The model under review builds one solid part; all positions refer to its coordinate system, in mm. Round coordinates to 2 decimals unless told otherwise and drop trailing zeros. Order: outer loops, then holes, each group sorted by start corner. A loop starts at its lowest first (then second) coordinate and runs counter-clockwise, first axis right, second up. Notation, with made-up numbers: M 76.5,-8 L 105.5,-8 A22 cw 105.5,21 Z; hole C 76,-8.5 d4. An arc over 180 degrees is marked long. Answer as a JSON object with one key per item and string values. Group by question number.
1. Add section C-C on x = -44. State the section outline as (y, z) points.
2. Add section A-A on z = 279.4. State the section outline as (x, y) points (3 decimals), and give its area (3 significant figures).
3. Clearance check with a flat-ended pin moving along its axis: P1, Ø17, axis at x = 0, z = 101.6, coming from the -Y side. State where the tip first meets the part, or that it passes through.
4. To check wall thickness, follow probe 1 along Z at (x, y) = (0, -13) (3 decimals); probe 2 along X at (y, z) = (6, 101); probe 3 along Z at (x, y) = (5, -22.5). State the ranges of each line that lie inside material, in increasing order. Write a range as [from, to].
5. Add section B-B on x = 0. State the section outline as (y, z) points (3 decimals).
6. Mouldability with a two-part tool opening along Z and no side actions: class faces 1 (the face through (-1, 0, 381)), 2 (the face through (-50.8, 0, 188)), 3 (the face through (-2.06, 0.36, 110.9)) as released by +Z, released by -Z, zero draft, split by the parting line, or undercut.
Autodesk Inventor part; units mm, degrees
ref_plane "YZ Plane" through (0, 0, 0) normal (1, 0, 0) x (0, 1, 0)
ref_plane "XZ Plane" through (0, 0, 0) normal (0, 1, 0) x (-1, 0, 0)
ref_plane "XY Plane" through (0, 0, 0) normal (0, 0, 1) x (1, 0, 0)
sketch "Sketch1" plane through (0, 0, 0) normal (0, 0, 1) x (1, 0, 0)
  line L0 (-38.1, -25.4) -> (38.1, -25.4)
  line L1 (50.8, -12.7) -> (50.8, 12.7)
  line L2 (38.1, 25.4) -> (-38.1, 25.4)
  line L3 (-50.8, 12.7) -> (-50.8, -12.7)
  line L4 (-50.8, -25.4) -> (50.8, 25.4) construction
  line L5 (50.8, -25.4) -> (-50.8, 25.4) construction
  arc A0 (-38.1, 25.4) -> (-50.8, 12.7) centre (-38.1, 12.7) ccw
  arc A1 (-50.8, -12.7) -> (-38.1, -25.4) centre (-38.1, -12.7) ccw
  arc A2 (38.1, -25.4) -> (50.8, -12.7) centre (38.1, -12.7) ccw
  arc A3 (50.8, 12.7) -> (38.1, 25.4) centre (38.1, 12.7) ccw
  point P0 (0, 0)
  dimension "d0" = 12.7
  dimension "d1" = 101.6
  dimension "d2" = 50.8
extrude "Extrusion1" add sketch "Sketch1" along normal blind 381
sketch "Sketch2" plane through (-38.1, 25.4, 0) normal (0, 1, 0) x (1, 0, 0)
  circle A0 centre (38.1, -279.4) radius 9.525
  circle A1 centre (38.1, -101.6) radius 9.525
  line L0 (-12.7, 0) -> (-12.7, -381)
  line L1 (76.2, 0) -> (0, 0)
  point P0 (38.1, 0)
  point P1 (-12.7, -190.5)
  point P2 (38.1, 0)
  dimension "d6" = 88.9
  dimension "d7" = 19.05
  dimension "d8" = 177.8
extrude "Extrusion2" cut sketch "Sketch2" against normal blind 381
properties part number "Wood-1"
Recorded:
{
 "1": {"outline": "M -23.95,0 L 23.95,0 L 23.95,381 L -23.95,381 Z"},
 "2": {"outline": "M -50.8,-12.7 A12.7 ccw -38.1,-25.4 L -9.525,-25.4 L -9.525,25.4 L -38.1,25.4 A12.7 ccw -50.8,12.7 Z; M 9.525,-25.4 L 38.1,-25.4 A12.7 ccw 50.8,-12.7 L 50.8,12.7 A12.7 ccw 38.1,25.4 L 9.525,25.4 Z", "area": "4,060 mm²"},
 "3": {"P1": "passes through"},
 "4": {"probe 1": "z = [0, 92.075], [111.125, 269.875], [288.925, 381]", "probe 2": "x = [-50.8, -9.51], [9.51, 50.8]", "probe 3": "z = [0, 93.49], [109.71, 271.29], [287.51, 381]"},
 "5": {"outline": "M -25.4,0 L 25.4,0 L 25.4,92.075 L -25.4,92.075 Z; M -25.4,111.125 L 25.4,111.125 L 25.4,269.875 L -25.4,269.875 Z; M -25.4,288.925 L 25.4,288.925 L 25.4,381 L -25.4,381 Z"},
 "6": {"face 1": "released by +Z", "face 2": "zero draft", "face 3": "undercut"}
}
